Verification items for the finished model (mm, model axes). Face numbers are marked on the shaded views. Give positions to 0.01 mm unless a question says otherwise; leave off trailing zeros. Order: outer loops, then holes, each group sorted by start corner. A loop starts at its lowest first (then second) coordinate and runs counter-clockwise, first axis right, second up.
(1) Sectioned sample at D-D on z = 0.8. Record the cut outline in (x, y).
(2) Sectioned sample at A-A on z = 2. Record the cut outline in (x, y), plus the area to 3 significant figures.
(3) Sectioned sample at C-C on x = 0.5. Record the cut outline in (y, z).
(4) Gauge pin test, flat ends, axial feed: pin 1 (3 mm diameter, centred on x = 0.5, y = 8, fed in from -Z); pin 2 (1 mm diameter, centred on y = -1.5, z = 0.5, fed in from -X). Record the tip position at first contact, or that the pin passes through.
(5) Sectioned sample at B-B on y = 8. Record the cut outline in (x, z), plus the area to 3 significant figures.
(6) Mould release check, pull along Y, two halves, no side actions. Record for the marked faces 1, 2 and 3: pulls with the +Y half, pulls with the -Y half, needs draft (parallel to the pull), parting line crosses it, or undercut.
(7) Scan lines: L1, parallel to Y at x = 0.5, z = 0.35; L2, parallel to Y at x = -6.25, z = 2.35; L3, parallel to Y at x = 1.5, z = 0.95. Record each from-to range of solid material in increasing order.
```python
from build123d import *

# Parameters (mm, degrees)
SKETCH_1_W             = 10
SKETCH_1_H             = 25
SKETCH_1_R             = 1.75
EXTRUDE_1_DEPTH        = 1.2
SKETCH_3_R             = 2
EXTRUDE_3_DEPTH        = 6
PATTERN_LINEAR_2_COUNT = 2
PATTERN_LINEAR_2_PITCH = 14


with BuildPart() as part:
    # 草图1 → 凸台-拉伸1 (new body)
    with BuildSketch(Plane.XY):
        Rectangle(SKETCH_1_W, SKETCH_1_H)
        with Locations((0.5, 8)):
            Circle(SKETCH_1_R, mode=Mode.SUBTRACT)
        with Locations((0.5, -8)):
            Circle(SKETCH_1_R, mode=Mode.SUBTRACT)
    extrude(amount=EXTRUDE_1_DEPTH)

    # 草图3 → 凸台-拉伸3 (add)
    with BuildSketch(Plane.XZ.offset(12.5)):
        with Locations((-5, 2)):
            Circle(SKETCH_3_R)
    extrude_3 = extrude(amount=-EXTRUDE_3_DEPTH)

    # 阵列(线性)2: 凸台-拉伸3 ×2
    with Locations(*[(0, i * PATTERN_LINEAR_2_PITCH, 0) for i in range(1, PATTERN_LINEAR_2_COUNT)]):
        add(extrude_3)


solid = part.part
```
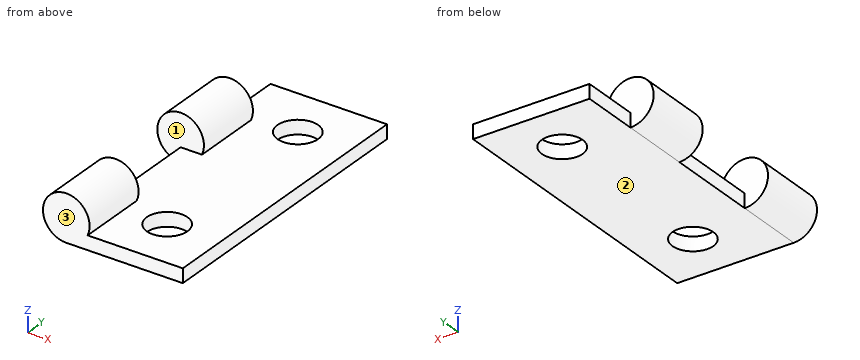
Ans:
1. outline: (-6.6, -12.5) - (5, -12.5) - (5, 12.5) - (-5, 12.5) - (-5, 7.5) - (-6.6, 7.5) - (-6.6, 1.5) - (-5, 1.5) - (-5, -6.5) - (-6.6, -6.5) - close; hole circle Ø3.5 at (0.5, -8); hole circle Ø3.5 at (0.5, 8)
2. outline: (-7, -12.5) - (-3, -12.5) - (-3, -6.5) - (-7, -6.5) - close; (-7, 1.5) - (-3, 1.5) - (-3, 7.5) - (-7, 7.5) - close
2. area: 48.0 mm2
3. outline: (-12.5, 0) - (-9.75, 0) - (-9.75, 1.2) - (-12.5, 1.2) - close; (-6.25, 0) - (6.25, 0) - (6.25, 1.2) - (-6.25, 1.2) - close; (9.75, 0) - (12.5, 0) - (12.5, 1.2) - (9.75, 1.2) - close
4. pin 1: passes through
4. pin 2: stops at x = -5
5. outline: (-5, 0) - (-1.25, 0) - (-1.25, 1.2) - (-5, 1.2) - close; (2.25, 0) - (5, 0) - (5, 1.2) - (2.25, 1.2) - close
5. area: 7.80 mm2
6. face 1: undercut
6. face 2: needs draft
6. face 3: pulls with the -Y half
7. L1: y = -12.5 to -9.75, -6.25 to 6.25, 9.75 to 12.5
7. L2: y = -12.5 to -6.5, 1.5 to 7.5
7. L3: y = -12.5 to -9.44, -6.56 to 6.56, 9.44 to 12.5
